```python
from build123d import *

# Parameters (mm, degrees)
RESSALTO_EXTRUS_O1_DEPTH = 2.5
FILETE1_R                = 0.1


with BuildPart() as part:
    # Esboço1 → Ressalto-extrusão1 (new body)
    with BuildSketch(Plane.XY):
        with BuildLine():
            Line((-184.814110363, 146.520645343), (-184.814110363, 152.820645343))
            Line((-184.814110363, 152.820645343), (-182.314110363, 152.820645343))
            Line((-182.314110363, 152.820645343), (-182.314110363, 146.520645343))
            Line((-182.314110363, 146.520645343), (-141.314110363, 146.520645343))
            Line((-141.314110363, 146.520645343), (-141.314110363, 152.820645343))
            Line((-141.314110363, 152.820645343), (-138.814110363, 152.820645343))
            Line((-138.814110363, 152.820645343), (-138.814110363, 146.520645343))
            Line((-138.814110363, 146.520645343), (-131.014110363, 146.520645343))
            ThreePointArc((-131.014110363, 146.520645343), (-124.714110363, 152.820645343), (-131.014110363, 159.120645343))
            Line((-131.014110363, 159.120645343), (-192.614110363, 159.120645343))
            ThreePointArc((-192.614110363, 159.120645343), (-198.914110363, 152.820645343), (-192.614110363, 146.520645343))
            Line((-192.614110363, 146.520645343), (-184.814110363, 146.520645343))
        make_face()
    extrude(amount=RESSALTO_EXTRUS_O1_DEPTH)

    # Filete1
    filete1_edges = [part.edges().sort_by_distance(p)[0] for p in [
        (-124.714110363, 152.820645343, 2.5),
        (-138.814110363, 149.670645343, 0),
        (-140.064110363, 152.820645343, 0),
        (-141.314110363, 149.670645343, 0),
        (-161.814110363, 159.120645343, 2.5),
        (-161.814110363, 146.520645343, 0),
        (-182.314110363, 149.670645343, 0),
        (-183.564110363, 152.820645343, 0),
        (-184.814110363, 149.670645343, 0),
        (-188.714110363, 146.520645343, 0),
        (-198.914110363, 152.820645343, 0),
        (-161.814110363, 159.120645343, 0),
        (-124.714110363, 152.820645343, 0),
        (-198.914110363, 152.820645343, 2.5),
        (-134.914110363, 146.520645343, 0),
        (-138.814110363, 146.520645343, 1.25),
        (-138.814110363, 152.820645343, 1.25),
        (-141.314110363, 152.820645343, 1.25),
        (-141.314110363, 146.520645343, 1.25),
        (-182.314110363, 146.520645343, 1.25),
        (-182.314110363, 152.820645343, 1.25),
        (-184.814110363, 152.820645343, 1.25),
        (-184.814110363, 146.520645343, 1.25),
        (-188.714110363, 146.520645343, 2.5),
        (-184.814110363, 149.670645343, 2.5),
        (-183.564110363, 152.820645343, 2.5),
        (-182.314110363, 149.670645343, 2.5),
        (-161.814110363, 146.520645343, 2.5),
        (-141.314110363, 149.670645343, 2.5),
        (-134.914110363, 146.520645343, 2.5),
        (-140.064110363, 152.820645343, 2.5),
        (-138.814110363, 149.670645343, 2.5),
    ]]
    fillet(filete1_edges, radius=FILETE1_R)


solid = part.part
```
Could you check a few things on this model? Use its own coordinates, in mm. A direction names the side the tool comes from. Give positions to 0.01 mm unless a question says otherwise; leave off trailing zeros. Loops run counter-clockwise (first coordinate to the right, second up) from the corner with the lowest first, then second, coordinate; pieces in that order, holes last. Notation, with made-up numbers: (-12.5, -33.75) - (0.5, -33.75) arc R25 ccw to (0.5, -3.75) - close; hole circle Ø2 at (30, 69.25). An arc over 180 degrees is marked (long way). Use one line per item in the form item = value.
1. I want a section at A-A (z = 1.65). Please give me the cut outline in (x, y), and give its area (3 significant figures).
Response values:
outline = (-192.61, 146.52) - (-184.91, 146.52) arc R0.1 ccw to (-184.81, 146.62) - (-184.81, 152.72) arc R0.1 cw to (-184.71, 152.82) - (-182.41, 152.82) arc R0.1 cw to (-182.31, 152.72) - (-182.31, 146.62) arc R0.1 ccw to (-182.21, 146.52) - (-141.41, 146.52) arc R0.1 ccw to (-141.31, 146.62) - (-141.31, 152.72) arc R0.1 cw to (-141.21, 152.82) - (-138.91, 152.82) arc R0.1 cw to (-138.81, 152.72) - (-138.81, 146.62) arc R0.1 ccw to (-138.71, 146.52) - (-131.01, 146.52) arc R6.3 ccw to (-131.01, 159.12) - (-192.61, 159.12) arc R6.3 ccw to start
area = 869 mm²
2. Thinking about a two-plate mould opening in X: for faces 1 (the face through (-162, 153, 2.5)), 2 (the face through (-182.314, 150, 1)), 3 (the face through (-198.913, 152.959, 1.234)), 4 (the face through (-124.716, 152.682, 1.234)), which applies, released by +X, released by -X, zero draft, split by the parting line, or undercut?
Response values:
face_1 = zero draft
face_2 = undercut
face_3 = released by -X
face_4 = released by +X
3. I need wall thicknesses on probe 1 along X at (y, z) = (151.75, 2.2); probe 2 along X at (y, z) = (150, 0.65); probe 3 along X at (y, z) = (153.25, 2.15). Which ranges of each line are inside material? Lowest first, please.
Response values:
probe_1 = -198.82 to -184.81, -182.31 to -141.31, -138.81 to -124.81
probe_2 = -198.25 to -184.81, -182.31 to -141.31, -138.81 to -125.38
probe_3 = -198.9 to -124.73
4. On a 3-axis mill with a long thin cutter (end or side, diameter ignored), from which of +Z, -Z, +X, -X, +Y, -Y can I reach the whole of each face in a straight line? I mean faces 5 (the face through (-141.314, 150, 1)), 6 (the face through (-135, 146.521, 1)). Say none if no direction works.
Response values:
face_5 = +Z, -Z, -Y
face_6 = +Z, -Z, +X, -X, -Y
5. I'm going to push flat-ended pins straight in: pin 1 Ø0.7 at (y, z) = (149, 1.5) entering from -X; pin 2 Ø1.2 at (x, z) = (-183.5, 1) entering from -Y; pin 3 Ø1.2 at (y, z) = (149, 2) entering from -X. Where does each tip first touch, or does it pass through?
Response values:
pin_1 = -197.87
pin_2 = 152.82
pin_3 = -198.03
6. I want a section at C-C (y = 151). Give the number of separate pieces and of enclosed holes in the cut face, and give its area (3 significant figures).
Response values:
separate_pieces = 3
enclosed_holes = 0
area = 172 mm²
7. I want a section at B-B (x = -140). Please give me the cut outline in (y, z), and give its area (3 significant figures).
Response values:
outline = (152.82, 0.1) arc R0.1 ccw to (152.92, 0) - (159.02, 0) arc R0.1 ccw to (159.12, 0.1) - (159.12, 2.4) arc R0.1 ccw to (159.02, 2.5) - (152.92, 2.5) arc R0.1 ccw to (152.82, 2.4) - close
area = 15.7 mm²
